from build123d import *

# Parameters (mm, degrees)
F0_W     = 88
F0_H     = 130
F0_R     = 4
F0_R_2   = 3
F0_W_2   = 4
F0_H_2   = 47
F1_DEPTH = 4


with BuildPart() as f1:
    # F0 (on Front) → F1 (new body)
    with BuildSketch(Plane.XZ):
        with Locations((44, 65)):
            Rectangle(F0_W, F0_H)
        with Locations((11.5, 14)):
            Circle(F0_R, mode=Mode.SUBTRACT)
        with Locations((65, 6)):
            Circle(F0_R_2, mode=Mode.SUBTRACT)
        with Locations((82, 32.75)):
            Rectangle(F0_W_2, F0_H_2, mode=Mode.SUBTRACT)
        with Locations((11.5, 114)):
            Circle(F0_R, mode=Mode.SUBTRACT)
        with Locations((53.5, 73.5)):
            Rectangle(F0_W_2, F0_H_2, mode=Mode.SUBTRACT)
        with Locations((65, 124)):
            Circle(F0_R_2, mode=Mode.SUBTRACT)
    extrude(amount=F1_DEPTH)


solid = f1.part
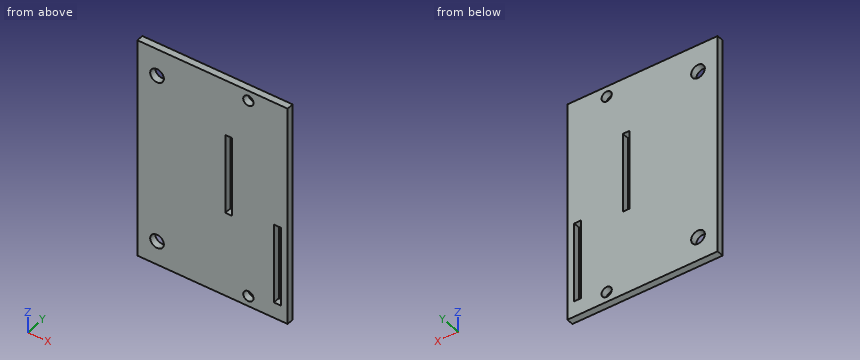
Design review of the part built by this model. Coordinates are the model's own, in mm. Coordinates: 2 decimals unless noted, no trailing zeros. Write each loop counter-clockwise with the first axis right and the second up, starting at its lowest first coordinate (ties: lowest second). Pieces come first, ordered by that corner, then holes. Notation, with made-up numbers: (-1, 18) -> (35, 18) arc R34 cw to (35, 54) -> close; hole circle Ø7 at (64, -11.75). An arc over 180 degrees is marked (long way). Write each question's results on one line, items separated by ' | '. Start each with the question number.
(1) Take a section at A-A on x = 11.5. Write out the cut boundary in (y, z).
(2) For line 1 along Z through (x, y) = (11.5, -1.9); line 2 along Z through (x, y) = (65, -2.5); line 3 along X through (y, z) = (-2.6, 42.5), list the stretches that pass through material, from the lowest coordinate up. Write a range as from..to.
(3) Take a section at C-C on y = -2. Write out the cut boundary in (x, z), and give its area (3 significant figures).
(4) Take a section at D-D on z = 14. Write out the cut boundary in (x, y).
(5) Take a section at B-B on z = 124. Write out the cut boundary in (x, y), and give its area (3 significant figures).
(6) Clearance check with a flat-ended pin moving along its axis: P1, Ø5, axis at x = 65, z = 6, coming from the -Y side. State where the tip first meets the part, or that it passes through.
Results found:
1) outline: (-4, 0) -> (0, 0) -> (0, 10) -> (-4, 10) -> close; (-4, 18) -> (0, 18) -> (0, 110) -> (-4, 110) -> close; (-4, 118) -> (0, 118) -> (0, 130) -> (-4, 130) -> close
2) line 1: z = 0..10, 18..110, 118..130 | line 2: z = 0..3, 9..121, 127..130 | line 3: x = 0..80, 84..88
3) outline: (0, 0) -> (88, 0) -> (88, 130) -> (0, 130) -> close; hole circle Ø8 at (11.5, 14); hole circle Ø8 at (11.5, 114); hole (51.5, 50) -> (55.5, 50) -> (55.5, 97) -> (51.5, 97) -> close; hole circle Ø6 at (65, 6); hole circle Ø6 at (65, 124); hole (80, 9.25) -> (84, 9.25) -> (84, 56.25) -> (80, 56.25) -> close | area: 10,900 mm2
4) outline: (0, -4) -> (7.5, -4) -> (7.5, 0) -> (0, 0) -> close; (15.5, -4) -> (80, -4) -> (80, 0) -> (15.5, 0) -> close; (84, -4) -> (88, -4) -> (88, 0) -> (84, 0) -> close
5) outline: (0, -4) -> (62, -4) -> (62, 0) -> (0, 0) -> close; (68, -4) -> (88, -4) -> (88, 0) -> (68, 0) -> close | area: 328 mm2
6) P1: passes through
